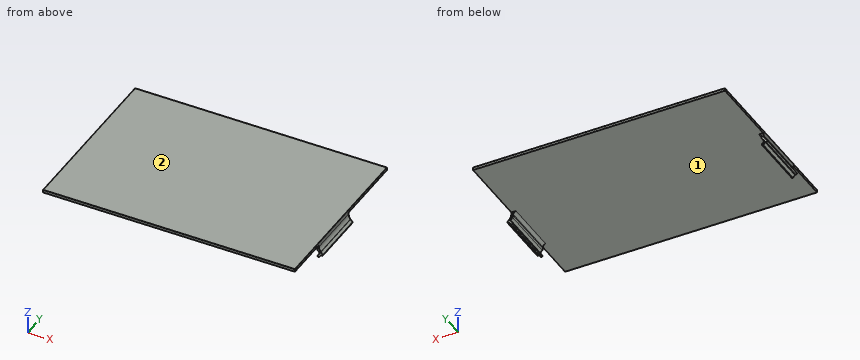
```python
from build123d import *

# Parameters (mm, degrees)
STOCK_OUTTER_CASE_1_START     = -135
STOCK_OUTTER_CASE_1_OUTLINE_W = 184.8
STOCK_OUTTER_CASE_1_OUTLINE_H = 3
STOCK_OUTTER_CASE_1_DEPTH     = 270
FILLET1_R                     = 0.2
BOSS_EXTRUDE1_DEPTH           = 29.8
FILLET2_R                     = 3
FILLET2_OF_MIRROR1_R          = 3
BOSS_EXTRUDE2_DEPTH           = 59.6
FILLET3_R                     = 0.5


# Read off the part's stored shape, not the designer's step: Stock-outter_case-1
with BuildPart() as part:
    # Stock-outter_case-1 outline → Stock-outter_case-1 (new body)
    with BuildSketch(Plane.YZ.offset(STOCK_OUTTER_CASE_1_START)):
        with Locations((88.4, 94.5)):
            Rectangle(STOCK_OUTTER_CASE_1_OUTLINE_W, STOCK_OUTTER_CASE_1_OUTLINE_H)
    extrude(amount=STOCK_OUTTER_CASE_1_DEPTH)

    # Fillet1
    fillet1_edges = [part.edges().sort_by_distance(p)[0] for p in [
        (0, 180.8, 96),
        (0, -4, 96),
        (135, 88.4, 96),
        (-135, 88.4, 96),
    ]]
    fillet(fillet1_edges, radius=FILLET1_R)

    # Sketch2 → Boss-Extrude1 (add, symmetric)
    with BuildSketch(Plane(origin=(0, 74, 0), x_dir=(1, 0, 0), z_dir=(0, 1, 0))):
        with BuildLine():
            Line((133, -93), (135, -93))
            Line((135, -93), (135, -91.139702343))
            ThreePointArc((135, -91.139702343), (135.482459034, -88.403541196), (136.871644455, -85.997401465))
            Line((136.871644455, -85.997401465), (137.206664088, -85.598140613))
            ThreePointArc((137.206664088, -85.598140613), (137.908530759, -83.669777784), (137.206664088, -81.741414955))
            Line((137.206664088, -81.741414955), (135.149743737, -79.290072737))
            ThreePointArc((135.149743737, -79.290072737), (134.606632777, -79.007347067), (134.022678095, -79.191467271))
            Line((134.022678095, -79.191467271), (133.716260318, -79.448582314))
            ThreePointArc((133.716260318, -79.448582314), (133.433534647, -79.991693275), (133.617654851, -80.575647957))
            Line((133.617654851, -80.575647957), (135.674575202, -83.026990175))
            ThreePointArc((135.674575202, -83.026990175), (135.908530759, -83.669777784), (135.674575202, -84.312565394))
            Line((135.674575202, -84.312565394), (133.701866671, -86.663547874))
            ThreePointArc((133.701866671, -86.663547874), (133.180922138, -87.565850273), (133, -88.591910703))
            Line((133, -88.591910703), (133, -93))
        make_face()
    boss_extrude1 = extrude(amount=BOSS_EXTRUDE1_DEPTH, both=True)

    # Fillet2
    fillet2_edges = [part.edges().sort_by_distance(p)[0] for p in [
        (133, 74, 93),
    ]]
    fillet(fillet2_edges, radius=FILLET2_R)

    # Mirror1: Boss-Extrude1 across plane
    add(boss_extrude1.mirror(Plane(origin=(0, 0, 0), x_dir=(0, 0, 1), z_dir=(1, 0, 0))))

    # Fillet2 of Mirror1
    fillet2_of_mirror1_edges = [part.edges().sort_by_distance(p)[0] for p in [
        (-133, 74, 93),
    ]]
    fillet(fillet2_of_mirror1_edges, radius=FILLET2_OF_MIRROR1_R)

    # Sketch3 → Boss-Extrude2 (add)
    with BuildSketch(Plane(origin=(0, 103.8, 0), x_dir=(1, 0, 0), z_dir=(0, 1, 0))):
        with BuildLine():
            Line((137.206664088, -85.598140613), (139.064378688, -83.384202565))
            ThreePointArc((139.064378688, -83.384202565), (139.204642032, -82.318796694), (138.298334245, -81.741414955))
            Line((138.298334245, -81.741414955), (137.206664088, -81.741414955))
            Line((137.206664088, -81.741414955), (137.206664088, -85.598140613))
        make_face()
    boss_extrude2 = extrude(amount=-BOSS_EXTRUDE2_DEPTH)

    # Mirror2: Boss-Extrude2 across plane
    add(boss_extrude2.mirror(Plane(origin=(0, 0, 0), x_dir=(0, 0, 1), z_dir=(1, 0, 0))))

    # Fillet3
    fillet3_edges = [part.edges().sort_by_distance(p)[0] for p in [
        (137.206664088, 74, 81.741414955),
        (-137.206664088, 74, 81.741414955),
    ]]
    fillet(fillet3_edges, radius=FILLET3_R)


solid = part.part
```
Work out the finished part from the listing and answer in its coordinate system (mm). Face numbers are marked on the shaded views. Coordinates: 2 decimals unless noted, no trailing zeros. Order: outer loops, then holes, each group sorted by start corner. A loop starts at its lowest first (then second) coordinate and runs counter-clockwise, first axis right, second up. Notation, with made-up numbers: M -28,47 L 11,47 A13 cw 11,68 Z; hole C 66.25,-36 d2. An arc over 180 degrees is marked long. Use CSV: the item, a comma, the result in double quotes.
1) Flat-ended cylindrical pins translate along their axes: pin 1 Ø7.5 at (x, z) = (-136, 84) entering from +Y; pin 2 Ø10 at (x, z) = (137, 87) entering from -Y; pin 3 Ø3 at (y, z) = (76.5, 92) entering from +X. Find the tip coordinate at first contact, or state that the pin passes through.
Worked out:
pin 1,"stops at y = 103.8"
pin 2,"stops at y = 44.2"
pin 3,"stops at x = 135.03"
2) Determine the mould class of the marked faces 1 and 2 for opening direction X: released by +X, released by -X, zero draft, split by the parting line, or undercut.
Worked out:
face 1,"undercut"
face 2,"zero draft"
3) Section A-A on x = -84.5 is taken. Write down the section's boundary in (y, z), plus the area to 3 significant figures.
Worked out:
outline,"M -4,93 L 180.8,93 L 180.8,95.8 A0.2 ccw 180.6,96 L -3.8,96 A0.2 ccw -4,95.8 Z"
area,"554 mm^2"
4) Section B-B on y = 17 is taken. Write down the section's boundary in (x, z).
Worked out:
outline,"M -135,93 L 135,93 L 135,95.8 A0.2 ccw 134.8,96 L -134.8,96 A0.2 ccw -135,95.8 Z"
5) Consider line 1 (Z direction, x = 44, y = 7); line 2 (X direction, y = 91, z = 83.5); line 3 (X direction, y = 149.5, z = 93.75). Determine where each line is inside the solid, lowest interval first. Write a range as [from, to].
Worked out:
line 1,"z = [93, 96]"
line 2,"x = [-138.97, -135.89], [135.89, 138.97]"
line 3,"x = [-135, 135]"
